from build123d import *

# Parameters (mm, degrees)
SKETCH2_W           = 160
SKETCH2_H           = 160
BOSS_EXTRUDE1_DEPTH = 2
SKETCH4_W           = 2
SKETCH4_H           = 160
BOSS_EXTRUDE3_DEPTH = 20
SKETCH5_W           = 180
SKETCH5_H           = 160
SKETCH5_W_2         = 176
SKETCH5_H_2         = 156
BOSS_EXTRUDE5_DEPTH = 100
SKETCH6_W           = 180
SKETCH6_H           = 160
SKETCH6_W_2         = 176
SKETCH6_H_2         = 156
BOSS_EXTRUDE6_DEPTH = 10


with BuildPart() as part:
    # Sketch2 → Boss-Extrude1 (new body)
    with BuildSketch(Plane.XY):
        Rectangle(SKETCH2_W, SKETCH2_H)
    extrude(amount=BOSS_EXTRUDE1_DEPTH)

    # Sketch4 → Boss-Extrude3 (add)
    with BuildSketch(Plane(origin=(80, 0, 0), x_dir=(0, 0, -1), z_dir=(1, 0, 0))):
        with Locations((-1, 0)):
            Rectangle(SKETCH4_W, SKETCH4_H)
    extrude(amount=BOSS_EXTRUDE3_DEPTH)

    # Sketch5 → Boss-Extrude5 (add)
    with BuildSketch(Plane.XY.offset(2)):
        with Locations((10, 0)):
            Rectangle(SKETCH5_W, SKETCH5_H)
        with Locations((10, 0)):
            Rectangle(SKETCH5_W_2, SKETCH5_H_2, mode=Mode.SUBTRACT)
    extrude(amount=BOSS_EXTRUDE5_DEPTH)

    # Sketch6 → Boss-Extrude6 (add)
    with BuildSketch(Plane.XY.offset(102)):
        with Locations((10, 0)):
            Rectangle(SKETCH6_W, SKETCH6_H)
        with Locations((10, 0)):
            Rectangle(SKETCH6_W_2, SKETCH6_H_2, mode=Mode.SUBTRACT)
    extrude(amount=BOSS_EXTRUDE6_DEPTH)


solid = part.part
Geometry: final body of the model. Coordinates: model frame, mm. A direction names the side the tool comes from. Give positions to 0.01 mm unless a question says otherwise; leave off trailing zeros. Write each loop counter-clockwise with the first axis right and the second up, starting at its lowest first coordinate (ties: lowest second). Pieces come first, ordered by that corner, then holes.
(1) Cut plane A-A, the plane z = 67.5. Return loops of the section in (x, y), then the cut area to 3 significant figures.
(2) Access query for faces 1 (the flat face through (9, -1, 2)), 2 (the flat face through (9, 80, 55)). Directions: +Z, -Z, +X, -X, +Y, -Y. A direction counts if a zero-diameter tool reaches every point of the face in a straight line with its end or side. Return the directions, or none.
(3) Cut plane C-C, the plane y = -11. Return loops of the section in (x, z).
(4) Cut plane B-B, the plane x = -24. Return loops of the section in (y, z), then the cut area to 3 significant figures.
(5) Mould query, pull axis X, two halves, no side actions, for faces 3 (the flat face through (100, -1, 55)), 4 (the flat face through (-80, -1, 55)), 5 (the flat face through (-78, -1, 56)), 6 (the flat face through (9, 78, 56)). Classes: released by +X, released by -X, zero draft, split by the parting line, or undercut.
(6) First-contact query: P1, Ø2, axis at x = 50.5, y = -25, coming from the +Z side. Flat tip, straight axial feed; report the tip coordinate or a pass-through.
(7) Ray query, line 1 (Y direction, x = 85.5, z = 19.5); line 2 (X direction, y = 40.5, z = 49); line 3 (Z direction, x = -5, y = -50.5). Return the intervals inside material, ascending.
Values follow:
1. outline: (-80, -80) - (100, -80) - (100, 80) - (-80, 80) - close; hole (-78, -78) - (98, -78) - (98, 78) - (-78, 78) - close
1. area: 1,340 mm2
2. face 1: +Z
2. face 2: +Z, -Z, +X, -X, +Y
3. outline: (-80, 0) - (100, 0) - (100, 112) - (98, 112) - (98, 2) - (-78, 2) - (-78, 112) - (-80, 112) - close
4. outline: (-80, 0) - (80, 0) - (80, 112) - (78, 112) - (78, 2) - (-78, 2) - (-78, 112) - (-80, 112) - close
4. area: 760 mm2
5. face 3: released by +X
5. face 4: released by -X
5. face 5: undercut
5. face 6: undercut
6. P1: stops at z = 2
7. line 1: y = -80 to -78, 78 to 80
7. line 2: x = -80 to -78, 98 to 100
7. line 3: z = 0 to 2
